CAD build for the part. Positions are in the model's coordinates, mm. A direction names the side the tool comes from. Coordinates: 2 decimals unless noted, no trailing zeros. Loops run counter-clockwise (first coordinate to the right, second up) from the corner with the lowest first, then second, coordinate; pieces in that order, holes last.
1) Wall check: line 1 along Z through (x, y) = (38, 11); line 2 along Y through (x, z) = (-54.5, 55.5); line 3 along X through (y, z) = (19.5, -54.5). Give the ranges that are in metal, low to high.
2) Pin check, flat tips, straight feed: pin 1 Ø8 at (y, z) = (30, 43.5) entering from +X; pin 2 Ø1.5 at (y, z) = (-33, -35.5) entering from -X; pin 3 Ø8 at (x, z) = (9.5, -40) entering from +Y. Stop position of each tip, or through.
3) Saw through at B-B, the plane x = -47. Write the cut outline in (y, z), and give its area (3 significant figures).
4) Saw through at A-A, the plane z = 3.5. Write the cut outline in (x, y).
5) Saw through at C-C, the plane y = -22. Write the cut outline in (x, z).
6) Which spindle directions (+Z, -Z, +X, -X, +Y, -Y) get a long thin tool onto all of the face, cutting with end or side? Do faces 1 (the flat face through (32, 22, -58.674)), 2 (the flat face through (-27, -1, -60.108)), 3 (the flat face through (32, 22, 0)), 4 (the flat face through (49, 0, -29)). Say none if no direction does.
```python
from build123d import *

# Parameters (mm, degrees)
F3_DEPTH = 58.674


with BuildPart() as f1:
    # F0 (on Front) → F1 (revolve)
    with BuildSketch(Plane.XZ):
        Polygon((27.523137, 37.01387), (27.523137, 60.107984), (-27.523137, 60.107984), (-27.523137, -60.107984), (27.523137, -60.107984), (27.523137, -54.729901), align=None)
    revolve(axis=Axis((-27.523137, 0, 0), (0, 0, -1)))

    # F2 (on Top) → F3 (join)
    with BuildSketch(Plane.XY):
        with BuildLine():
            Line((0, 0), (71.496874, 0))
            add(Edge.make_bspline(
                [(71.496874, 0), (30.049184, 17.29304), (23.930628, 55.467509), (-13.312755, 53.206302)],
                knots=[0, 0, 0, 0, 100.11785, 100.11785, 100.11785, 100.11785], degree=3))
            Line((-13.312755, 53.206302), (0, 0))
        make_face()
    extrude(amount=-F3_DEPTH)


solid = f1.part
```
Data:
1. line 1: z = -58.67 to 0
1. line 2: y = -47.98 to 47.98
1. line 3: x = -79 to 41.99
2. pin 1: stops at x = 21
2. pin 2: stops at x = -72.13
2. pin 3: stops at y = 50.34
3. outline: (-51.49, -60.11) - (51.49, -60.11) - (51.49, 60.11) - (-51.49, 60.11) - close
3. area: 12,400 mm2
4. outline: circle Ø110.09 at (-27.52, 0)
5. outline: (-77.98, -60.11) - (22.94, -60.11) - (22.94, 60.11) - (-77.98, 60.11) - close
6. face 1: -Z, +X, +Y
6. face 2: -Z, +X, -X, +Y, -Y
6. face 3: +Z, +X, +Y
6. face 4: +Z, -Z, +X, -Y
